Work out the finished part from the listing and answer in its coordinate system (mm). Face numbers are marked on the shaded views. Coordinates: 2 decimals unless noted, no trailing zeros. Loops run counter-clockwise (first coordinate to the right, second up) from the corner with the lowest first, then second, coordinate; pieces in that order, holes last. Notation, with made-up numbers: (-26.75, 47.25) -> (20.25, 47.25) arc R23 ccw to (20.25, 61.25) -> close; hole circle Ø2 at (15.5, 39.25). An arc over 180 degrees is marked (long way). Answer as CSV lines item,"result".
```python
from build123d import *

# Parameters (mm, degrees)
SKETCH1_W           = 27
SKETCH1_H           = 50
SKETCH1_R           = 3
SKETCH1_R_2         = 2.5
BOSS_EXTRUDE1_DEPTH = 5
FILLET2_R           = 1


with BuildPart() as part:
    # Sketch1 → Boss-Extrude1 (new body)
    with BuildSketch(Plane.XY):
        Rectangle(SKETCH1_W, SKETCH1_H)
        with Locations((-6.582992823, 18)):
            Circle(SKETCH1_R, mode=Mode.SUBTRACT)
        with Locations((-6.582992823, 0)):
            Circle(SKETCH1_R, mode=Mode.SUBTRACT)
        with Locations((-6.582992823, -18)):
            Circle(SKETCH1_R, mode=Mode.SUBTRACT)
        with Locations((6.5, 18)):
            Circle(SKETCH1_R_2, mode=Mode.SUBTRACT)
        with Locations((6.5, 0)):
            Circle(SKETCH1_R_2, mode=Mode.SUBTRACT)
        with Locations((6.5, -18)):
            Circle(SKETCH1_R_2, mode=Mode.SUBTRACT)
    extrude(amount=BOSS_EXTRUDE1_DEPTH)

    # Fillet2
    fillet2_edges = [part.edges().sort_by_distance(p)[0] for p in [
        (-13.5, 0, 5),
        (0, -25, 5),
        (13.5, 0, 5),
        (0, -25, 0),
        (-13.5, 0, 0),
        (0, 25, 0),
        (13.5, 0, 0),
        (13.5, -25, 2.5),
        (-13.5, -25, 2.5),
        (-13.5, 25, 2.5),
        (13.5, 25, 2.5),
        (0, 25, 5),
    ]]
    fillet(fillet2_edges, radius=FILLET2_R)


solid = part.part
```
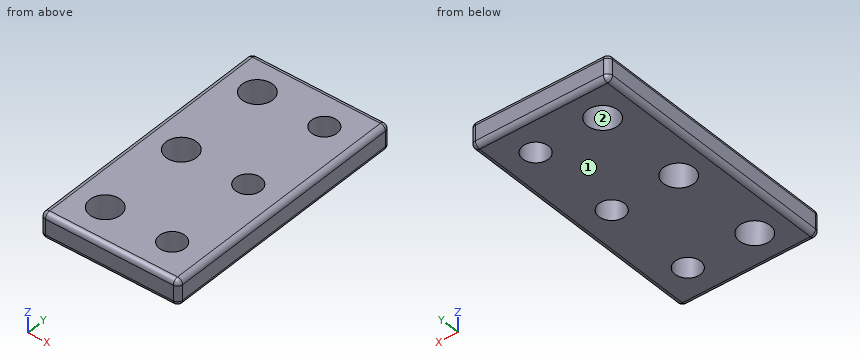
(1) For a pull along Y with two mould halves and no side action, classify the marked faces 1 and 2 as pulls with the +Y half, pulls with the -Y half, needs draft (parallel to the pull), parting line crosses it, or undercut.
Computed values:
face 1,"needs draft"
face 2,"undercut"
(2) A cutting plane is placed at B-B, the plane x = 6.5. Write down the section's boundary in (y, z), and give its area (3 significant figures).
Computed values:
outline,"(-25, 1) arc R1 ccw to (-24, 0) -> (-20.5, 0) -> (-20.5, 5) -> (-24, 5) arc R1 ccw to (-25, 4) -> close; (-15.5, 0) -> (-2.5, 0) -> (-2.5, 5) -> (-15.5, 5) -> close; (2.5, 0) -> (15.5, 0) -> (15.5, 5) -> (2.5, 5) -> close; (20.5, 0) -> (24, 0) arc R1 ccw to (25, 1) -> (25, 4) arc R1 ccw to (24, 5) -> (20.5, 5) -> close"
area,"174 mm2"
(3) Flat-ended cylindrical pins translate along their axes: pin 1 Ø5.5 at (x, y) = (-6.58, -18) entering from +Z (3 decimals); pin 2 Ø8 at (x, y) = (6.5, 0) entering from +Z. Find the tip coordinate at first contact, or state that the pin passes through.
Computed values:
pin 1,"through"
pin 2,"z = 5"
(4) A cutting plane is placed at A-A, the plane z = 2.25. Write down the section's boundary in (x, y).
Computed values:
outline,"(-13.5, -24) arc R1 ccw to (-12.5, -25) -> (12.5, -25) arc R1 ccw to (13.5, -24) -> (13.5, 24) arc R1 ccw to (12.5, 25) -> (-12.5, 25) arc R1 ccw to (-13.5, 24) -> close; hole circle Ø6 at (-6.58, -18); hole circle Ø6 at (-6.58, 0); hole circle Ø6 at (-6.58, 18); hole circle Ø5 at (6.5, -18); hole circle Ø5 at (6.5, 0); hole circle Ø5 at (6.5, 18)"
(5) A cutting plane is placed at C-C, the plane y = 0. Write down the section's boundary in (x, z), and give its area (3 significant figures).
Computed values:
outline,"(-13.5, 1) arc R1 ccw to (-12.5, 0) -> (-9.58, 0) -> (-9.58, 5) -> (-12.5, 5) arc R1 ccw to (-13.5, 4) -> close; (-3.58, 0) -> (4, 0) -> (4, 5) -> (-3.58, 5) -> close; (9, 0) -> (12.5, 0) arc R1 ccw to (13.5, 1) -> (13.5, 4) arc R1 ccw to (12.5, 5) -> (9, 5) -> close"
area,"79.1 mm2"
(6) Consider line 1 along Y through (x, z) = (6.5, 1.7); line 2 along Y through (x, z) = (-8.5, 0.7); line 3 along X through (y, z) = (-1, 2.7). Determine where each line is inside the solid, lowest interval first.
Computed values:
line 1,"-25 to -20.5, -15.5 to -2.5, 2.5 to 15.5, 20.5 to 25"
line 2,"-24.95 to -20.31, -15.69 to -2.31, 2.31 to 15.69, 20.31 to 24.95"
line 3,"-13.5 to -9.41, -3.75 to 4.21, 8.79 to 13.5"
(7) A cutting plane is placed at D-D, the plane y = -17. Write down the section's boundary in (x, z).
Computed values:
outline,"(-13.5, 1) arc R1 ccw to (-12.5, 0) -> (-9.41, 0) -> (-9.41, 5) -> (-12.5, 5) arc R1 ccw to (-13.5, 4) -> close; (-3.75, 0) -> (4.21, 0) -> (4.21, 5) -> (-3.75, 5) -> close; (8.79, 0) -> (12.5, 0) arc R1 ccw to (13.5, 1) -> (13.5, 4) arc R1 ccw to (12.5, 5) -> (8.79, 5) -> close"
